Part model, mm, in its own coordinate system. A direction names the side the tool comes from. Round coordinates to 2 decimals unless told otherwise and drop trailing zeros. Write each loop counter-clockwise with the first axis right and the second up, starting at its lowest first coordinate (ties: lowest second). Pieces come first, ordered by that corner, then holes. Notation, with made-up numbers: M -12.5,50 L 36.5,50 A14 cw 36.5,62 Z; hole C -15,-35 d9. An arc over 180 degrees is marked long. Answer as a JSON object with one key per item and string values. Group by question number.
1. Two-plate mould, pull along X, no slides. Class faces 3 (the face through (-11, 62.026, 6)), 4 (the face through (44, -55, 3)), 5 (the face through (49.756, 1, 6)): +X half, -X half, draft (parallel to the pull), parting line (faces both ways), or undercut.
2. Drop flat-ended pins along their axis: pin 1 (2.5 mm diameter, centred on x = -12, y = -8.5, fed in from +Z); pin 2 (10 mm diameter, centred on x = 16, y = -3.5, fed in from +Z). Give the stop position or say it passes through.
3. Band-saw the part on B-B, the plane x = -52. Write the cut outline in (y, z), plus the area to 3 significant figures.
4. Which spindle directions (+Z, -Z, +X, -X, +Y, -Y) get a long thin tool onto all of the face, cutting with end or side? Do faces 1 (the face through (-11, -57.974, 6)), 2 (the face through (-11, -5, 3)). Say none if no direction does.
5. Drill centre lines: line 1 (Y direction, x = -21, z = 10.5); line 2 (X direction, y = 33, z = 10.25); line 3 (Z direction, x = 13, y = 4). Where is each one in solid material? Low to high. Write a range as from..to.
6. Band-saw the part on A-A, the plane y = -26.5. Write the cut outline in (x, z), plus the area to 3 significant figures.
from build123d import *

# Parameters (mm, degrees)
SKETCH_1_W          = 120
SKETCH_1_H          = 120
EXTRUDE_1_DEPTH     = 12
SKETCH_2_W          = 104
SKETCH_2_H          = 91
CUT_EXTRUDE_1_DEPTH = 3
SKETCH_4_R          = 2.25
CUT_EXTRUDE_3_DEPTH = 12
SKETCH_6_R          = 1.75
CUT_EXTRUDE_5_DEPTH = 12
SKETCH_7_R          = 2.9
SKETCH_7_R_2        = 4.4
CUT_EXTRUDE_6_DEPTH = 9
SKETCH_8_R          = 1.5
CUT_EXTRUDE_7_DEPTH = 12


with BuildPart() as part:
    # 草图1 → 凸台-拉伸1 (new body)
    with BuildSketch(Plane.XY):
        with Locations((-10.243902439, 2.026266417)):
            Rectangle(SKETCH_1_W, SKETCH_1_H)
    extrude(amount=EXTRUDE_1_DEPTH)

    # 草图2 → 切除-拉伸1 (cut)
    with BuildSketch(Plane.XY.offset(12)):
        with Locations((-10.243902439, 11.360648518)):
            Rectangle(SKETCH_2_W, SKETCH_2_H)
    extrude(amount=-CUT_EXTRUDE_1_DEPTH, mode=Mode.SUBTRACT)

    # 草图4 → 切除-拉伸3 (cut)
    with BuildSketch(Plane.XY.offset(12)):
        with Locations((-10.243902439, -7.42403473)):
            Circle(SKETCH_4_R)
    extrude(amount=-CUT_EXTRUDE_3_DEPTH, mode=Mode.SUBTRACT)

    # 草图6 → 切除-拉伸5 (cut)
    with BuildSketch(Plane.XY.offset(12)):
        with Locations((-62.743902439, -53.42403473)):
            Circle(SKETCH_6_R)
        with Locations((42.256097561, -53.42403473)):
            Circle(SKETCH_6_R)
    extrude(amount=-CUT_EXTRUDE_5_DEPTH, mode=Mode.SUBTRACT)

    # 草图7 → 切除-拉伸6 (cut)
    with BuildSketch(Plane.XY.offset(12)):
        with Locations((-62.743902439, -53.42403473)):
            Circle(SKETCH_7_R)
        with Locations((42.256097561, -53.42403473)):
            Circle(SKETCH_7_R)
        with Locations((-10.243902439, -7.42403473)):
            Circle(SKETCH_7_R_2)
    extrude(amount=-CUT_EXTRUDE_6_DEPTH, mode=Mode.SUBTRACT)

    # 草图8 → 切除-拉伸7 (cut)
    with BuildSketch(Plane.XY.offset(12)):
        with Locations((-64.743902439, -18.139351482)):
            Circle(SKETCH_8_R)
        with Locations((-64.743902439, 41.860648518)):
            Circle(SKETCH_8_R)
        with Locations((44.256097561, 41.860648518)):
            Circle(SKETCH_8_R)
        with Locations((44.256097561, -18.139351482)):
            Circle(SKETCH_8_R)
    extrude(amount=-CUT_EXTRUDE_7_DEPTH, mode=Mode.SUBTRACT)


solid = part.part
Worked answers:
{
 "1": {"face 3": "draft", "face 4": "undercut", "face 5": "+X half"},
 "2": {"pin 1": "stops at z = 3", "pin 2": "stops at z = 9"},
 "3": {"outline": "M -57.97,0 L 62.03,0 L 62.03,12 L 56.86,12 L 56.86,9 L -34.14,9 L -34.14,12 L -57.97,12 Z", "area": "1,170 mm^2"},
 "4": {"face 1": "+Z, -Z, +X, -X, -Y", "face 2": "+Z"},
 "5": {"line 1": "y = -57.97..-34.14, 56.86..62.03", "line 2": "x = -70.24..-62.24, 41.76..49.76", "line 3": "z = 0..9"},
 "6": {"outline": "M -70.24,0 L 49.76,0 L 49.76,12 L 41.76,12 L 41.76,9 L -62.24,9 L -62.24,12 L -70.24,12 Z", "area": "1,130 mm^2"}
}
